The model under review builds one solid part; all positions refer to its coordinate system, in mm. Face numbers are marked on the shaded views. A direction names the side the tool comes from. Coordinates: 2 decimals unless noted, no trailing zeros. Order: outer loops, then holes, each group sorted by start corner. A loop starts at its lowest first (then second) coordinate and runs counter-clockwise, first axis right, second up. Notation, with made-up numbers: M -6,67 L 34,67 A26 cw 34,98 Z; hole C 9.5,8 d10. An arc over 180 degrees is marked long. Answer in a Markdown table with one row per item.
from build123d import *

# Parameters (mm, degrees)
SKETCH1_R           = 15
BOSS_EXTRUDE1_DEPTH = 75
CUT_EXTRUDE1_DEPTH  = 52
CUT_EXTRUDE2_DEPTH  = 3.5
SKETCH9_R           = 10
CUT_EXTRUDE12_DEPTH = 70
SKETCH17_W          = 7
SKETCH17_H          = 12
CUT_EXTRUDE19_DEPTH = 15
SKETCH19_W          = 7
SKETCH19_H          = 12
CUT_EXTRUDE20_DEPTH = 15


with BuildPart() as part:
    # Sketch1 → Boss-Extrude1 (new, symmetric)
    with BuildSketch(Plane(origin=(0, 0, 0), x_dir=(1, 0, 0), z_dir=(0, 1, 0))):
        with Locations(Location((0, 0, 0), (0, 0, 270))):
            Circle(SKETCH1_R)
    extrude(amount=BOSS_EXTRUDE1_DEPTH, both=True)

    # Sketch2 → Cut-Extrude1 (cut)
    with BuildSketch(Plane.XZ.offset(75)):
        with BuildLine():
            Line((3.5, 15), (3.5, -15))
            ThreePointArc((3.5, -15), (0, -18.5), (-3.5, -15))
            Line((-3.5, -15), (-3.5, 15))
            ThreePointArc((-3.5, 15), (0, 18.5), (3.5, 15))
        make_face()
    extrude(amount=-CUT_EXTRUDE1_DEPTH, mode=Mode.SUBTRACT)

    # Sketch3 → Cut-Extrude2 (cut, symmetric)
    with BuildSketch(Plane(origin=(0, -26.5, 0), x_dir=(1, 0, 0), z_dir=(0, 1, 0))):
        Polygon((-14.980069936, 0), (-15.328117643, -9.993941304), (-0.348047707, -16.993941304), (0, -7), align=None)
        Polygon((15, 0), (0, 7), (0.348047707, 16.993941304), (15.348047707, 9.993941304), align=None)
    extrude(amount=CUT_EXTRUDE2_DEPTH, both=True, mode=Mode.SUBTRACT)

    # Sketch9 → Cut-Extrude12 (cut)
    with BuildSketch(Plane.XZ.offset(75)):
        with Locations(Location((0, 0, 0), (0, 0, 270))):
            Circle(SKETCH9_R)
    extrude(amount=-CUT_EXTRUDE12_DEPTH, mode=Mode.SUBTRACT)

    # Sketch17 → Cut-Extrude19 (cut)
    with BuildSketch(Plane(origin=(15, 0, 0), x_dir=(0, 0, -1), z_dir=(1, 0, 0))):
        with Locations((3.5, -29)):
            Rectangle(SKETCH17_W, SKETCH17_H)
    extrude(amount=-CUT_EXTRUDE19_DEPTH, mode=Mode.SUBTRACT)

    # Sketch19 → Cut-Extrude20 (cut)
    with BuildSketch(Plane.ZY.offset(15)):
        with Locations((3.5, -29)):
            Rectangle(SKETCH19_W, SKETCH19_H)
    extrude(amount=-CUT_EXTRUDE20_DEPTH, mode=Mode.SUBTRACT)


solid = part.part
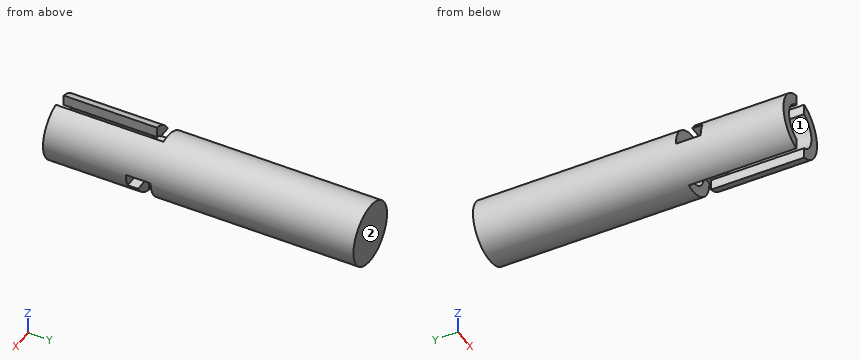
(1) Insertion check: P1, Ø2, axis at y = -17.5, z = 2, coming from the +X side; P2, Ø10, axis at x = 9.5, y = 6.5, coming from the -Z side; P3, Ø12, axis at x = 6.5, y = 54.5, coming from the -Z side. Each pin has a flat end and moves straight along its axis. Give the tip position at first contact, or say it passes through.
Report:
| item | result |
|---|---|
| P1 | x = 14.97 |
| P2 | z = -14.31 |
| P3 | z = -14.99 |
(2) Take a section at B-B (z = -4.25). Write out the cut boundary in (x, y), then the cut area to 3 significant figures.
Report:
| item | result |
|---|---|
| outline | M -14.39,-75 L -9.05,-75 L -9.05,-5 L 9.05,-5 L 9.05,-23 L 14.39,-23 L 14.39,75 L -14.39,75 Z; M 9.05,-75 L 14.39,-75 L 14.39,-35 L 9.05,-35 Z |
| area | 2,980 mm^2 |
(3) Machinability: for the marked faces 1 and 2, which of the approach directions +Z, -Z, +X, -X, +Y, -Y give a long, thin tool a straight path to every point of the face, cutting with its end or side? Answer none if there is none.
Report:
| item | result |
|---|---|
| face 1 | -Y |
| face 2 | +Z, -Z, +X, -X, +Y |
(4) To check wall thickness, follow line 1 (Y direction, x = -6.25, z = 12); line 2 (X direction, y = -20, z = 0); line 3 (Y direction, x = 1.5, z = -3.75). State the ranges of each line that lie inside material, in increasing order. Write a range as [from, to].
Report:
| item | result |
|---|---|
| line 1 | [-75, -30], [-23, 75] |
| line 2 | [-15, -10], [10, 15] |
| line 3 | [-5, 75] |
(5) Take a section at D-D (z = 3.75). Write out the cut boundary in (x, y), then the cut area to 3 significant figures.
Report:
| item | result |
|---|---|
| outline | M -14.52,-75 L -9.27,-75 L -9.27,-35 L -14.52,-35 Z; M -14.52,-23 L -9.27,-23 L -9.27,-5 L 9.27,-5 L 9.27,-75 L 14.52,-75 L 14.52,75 L -14.52,75 Z |
| area | 3,000 mm^2 |
(6) Take a section at A-A (x = 0). Write out the cut boundary in (y, z), then the cut area to 3 significant figures.
Report:
| item | result |
|---|---|
| outline | M -23,-15 L 75,-15 L 75,15 L -23,15 L -23,10 L -5,10 L -5,-10 L -23,-10 Z |
| area | 2,580 mm^2 |
(7) Take a section at C-C (y = 28). Write out the cut boundary in (x, z).
Report:
| item | result |
|---|---|
| outline | C 0,0 d30 |
